from build123d import *

# Parameters (mm, degrees)
BOSS_EXTRUDE1_DEPTH      = 2
BOSS_EXTRUDE1_DEPTH_BACK = 2
SKETCH3_R                = 1.75
BOSS_EXTRUDE2_START      = -2
BOSS_EXTRUDE2_DEPTH      = 4
CUT_EXTRUDE2_DEPTH       = 83.755664459


with BuildPart() as part:
    # Sketch3 → Boss-Extrude1 (new, two sides: drawn at the far end of the back side and taken through both)
    with BuildSketch(Plane.XY.offset(-BOSS_EXTRUDE1_DEPTH_BACK)):
        with BuildLine():
            Line((-12.648648649, -57.116212124), (-10.962162162, -49.500717174))
            Line((-10.962162162, -49.500717174), (-23.462338081, -45.092415448))
            ThreePointArc((-23.462338081, -45.092415448), (-26.50014347, -46.117965154), (-29.56784511, -45.185645238))
            ThreePointArc((-29.56784511, -45.185645238), (0, 49.5), (29.56784511, -45.185645238))
            ThreePointArc((29.56784511, -45.185645238), (26.50014347, -46.117965154), (23.462338081, -45.092415448))
            Line((23.462338081, -45.092415448), (10.962162162, -49.500717174))
            Line((10.962162162, -49.500717174), (12.648648649, -57.116212124))
            ThreePointArc((12.648648649, -57.116212124), (0, 58.5), (-12.648648649, -57.116212124))
        make_face()
        with Locations((-17.611521005, -49.939211163)):
            Circle(SKETCH3_R, mode=Mode.SUBTRACT)
        with Locations(Location((17.611521005, -49.939211163, 0), (0, 0, 180))):
            Circle(SKETCH3_R, mode=Mode.SUBTRACT)
    extrude(amount=BOSS_EXTRUDE1_DEPTH + BOSS_EXTRUDE1_DEPTH_BACK)

    # Sketch6 → Boss-Extrude2 (add)
    with BuildSketch(Plane.XY.offset(BOSS_EXTRUDE2_START)):
        with BuildLine():
            ThreePointArc((-24.625, 42.651751136), (0, 49.25), (24.625, 42.651751136))
            ThreePointArc((24.625, 42.651751136), (25.553522607, 42.616086127), (26.420381097, 42.28144814))
            ThreePointArc((26.420381097, 42.28144814), (0, 49.5), (-26.420381097, 42.28144814))
            ThreePointArc((-26.420381097, 42.28144814), (-25.553522607, 42.616086127), (-24.625, 42.651751136))
        make_face()
    extrude(amount=BOSS_EXTRUDE2_DEPTH)

    # Sketch5 → Cut-Extrude2 (cut, symmetric)
    with BuildSketch(Plane.XY):
        with BuildLine():
            Line((-23.462338081, -45.092415448), (0, 0))
            Line((0, 0), (-10.962162162, -49.500717174))
            ThreePointArc((-10.962162162, -49.500717174), (-17.295396026, -47.532334754), (-23.462338081, -45.092415448))
        make_face()
    cut_extrude2 = extrude(amount=CUT_EXTRUDE2_DEPTH, both=True, mode=Mode.SUBTRACT)

    # Mirror1: Cut-Extrude2 across plane
    add(cut_extrude2.mirror(Plane(origin=(0, 0, 0), x_dir=(0, 0, 1), z_dir=(1, 0, 0))), mode=Mode.SUBTRACT)


solid = part.part
Design review of the part built by this model. Coordinates are the model's own, in mm. A direction names the side the tool comes from. Coordinates: 2 decimals unless noted, no trailing zeros. Order: outer loops, then holes, each group sorted by start corner. A loop starts at its lowest first (then second) coordinate and runs counter-clockwise, first axis right, second up.
Item 1: For line 1 (X direction, y = -50, z = -1.75); line 2 (Y direction, x = -18, z = 1.2); line 3 (X direction, y = -42, z = 0.25), list the stretches that pass through material, from the lowest coordinate up.
Item 2: For pin 1 Ø2 at (x, z) = (37, -0.5) entering from -Y, flat-tipped, find the tip position at first contact; note if it passes through.
Item 3: Take a section at A-A, the plane y = 19. Write out the cut boundary in (x, z).
Item 4: Take a section at D-D, the plane x = 0. Write out the cut boundary in (y, z).
Item 5: The part is to be moulded in two halves that separate along X. For faces 4 (the flat face through (-13, 48, 2)), 5 (the cylindrical face through (2.39, 58.45, -0.03)), 6 (the cylindrical face through (-17.208, -47.563, 0.028)), say which applies: pulls with the +X half, pulls with the -X half, needs draft (parallel to the pull), parting line crosses it, or undercut.
Item 6: Take a section at B-B, the plane z = 1. Write out the cut boundary in (x, y) (3 decimals).
Item 7: For faces 1 (the flat face through (-13, 48, -2)), 2 (the cylindrical face through (51.895, 0.137, -0.028)), 3 (the flat face through (-11.817, -53.362, -0.028)), list the 3-axis set-ups (+Z, -Z, +X, -X, +Y, -Y) from which the entire face can be reached by the end or side of a thin tool; tool diameter is ignored.
Item 8: Take a section at C-C, the plane y = 0. Write out the cut boundary in (x, z).
The answers:
1. line 1: x = -30.37 to -19.36, -15.86 to -11.07, 11.07 to 15.86, 19.36 to 30.37
1. line 2: y = -55.66 to -51.65, -48.23 to -47.28, 45.84 to 55.66
1. line 3: x = -40.72 to -33.71, 33.71 to 40.72
2. pin 1: stops at y = -46.11
3. outline: (-55.33, -2) - (-47.32, -2) - (-47.32, 2) - (-55.33, 2) - close; (47.32, -2) - (55.33, -2) - (55.33, 2) - (47.32, 2) - close
4. outline: (49.25, -2) - (58.5, -2) - (58.5, 2) - (49.25, 2) - close
5. face 4: needs draft
5. face 5: parting line crosses it
5. face 6: undercut
6. outline: (-29.568, -45.186) arc R51.959 cw to (-26.42, 42.281) arc R2.828 cw to (-24.625, 42.652) arc R49.25 cw to (24.625, 42.652) arc R2.828 cw to (26.42, 42.281) arc R51.959 cw to (29.568, -45.186) arc R5.25 cw to (23.462, -45.092) arc R87.969 cw to (10.962, -49.501) - (12.649, -57.116) arc R58.5 ccw (long way) to (-12.649, -57.116) - (-10.962, -49.501) arc R87.969 cw to (-23.462, -45.092) arc R5.25 cw to start; hole circle Ø3.5 at (-17.612, -49.939); hole circle Ø3.5 at (17.612, -49.939)
7. face 1: -Z, +X, -X, +Y, -Y
7. face 2: +Z, -Z
7. face 3: +Z, -Z, -Y
8. outline: (-58.5, -2) - (-51.9, -2) - (-51.9, 2) - (-58.5, 2) - close; (51.9, -2) - (58.5, -2) - (58.5, 2) - (51.9, 2) - close
